```python
from build123d import *

# Parameters (mm, degrees)
F0_W      = 1625
F0_H      = 1960
F1_DEPTH  = 380
F2_W      = 920
F2_H      = 1960
F3_DEPTH  = 228
F4_W      = 1625
F4_H      = 645
F5_DEPTH  = 378
F6_W      = 1480
F6_H      = 185
F7_DEPTH  = 125
F9_DEPTH  = 2
F11_DEPTH = 1
F13_DEPTH = 25
F15_DEPTH = 1625.001


with BuildPart() as f1:
    # F0 (on Top) → F1 (new body)
    with BuildSketch(Plane.XY):
        with Locations((812.5, 980)):
            Rectangle(F0_W, F0_H)
    extrude(amount=F1_DEPTH)

    # F2 (on face) → F3 (cut)
    with BuildSketch(Plane.XY.offset(380)):
        with Locations((808, 980)):
            Rectangle(F2_W, F2_H)
    extrude(amount=-F3_DEPTH, mode=Mode.SUBTRACT)

    # F4 (on face) → F5 (cut)
    with BuildSketch(Plane.XY.offset(380)):
        with Locations((812.5, 1637.5)):
            Rectangle(F4_W, F4_H)
    extrude(amount=-F5_DEPTH, mode=Mode.SUBTRACT)

    # F6 (on face) → F7 (join)
    with BuildSketch(Plane.XY.offset(2)):
        with Locations((812.5, 1407.5)):
            Rectangle(F6_W, F6_H)
    extrude(amount=F7_DEPTH)

    # F8 (on face) → F9 (join)
    with BuildSketch(Plane(origin=(0, 1960, 0), x_dir=(-1, 0, 0), z_dir=(0, 1, 0))):
        with BuildLine():
            Line((-1625, 1126), (-1625, 0))
            Line((-1625, 0), (0, 0))
            Line((0, 0), (0, 1126))
            ThreePointArc((0, 1126), (-58.578644, 1267.421356), (-200, 1326))
            Line((-200, 1326), (-1425, 1326))
            ThreePointArc((-1425, 1326), (-1566.421356, 1267.421356), (-1625, 1126))
        make_face()
    extrude(amount=F9_DEPTH)

    # F10 (on face) → F11 (join)
    with BuildSketch(Plane.XZ):
        with BuildLine():
            Line((0, 1126), (0, 0))
            Line((0, 0), (1625, 0))
            Line((1625, 0), (1625, 1126))
            ThreePointArc((1625, 1126), (1566.421356, 1267.421356), (1425, 1326))
            Line((1425, 1326), (200, 1326))
            ThreePointArc((200, 1326), (58.578644, 1267.421356), (0, 1126))
        make_face()
    extrude(amount=F11_DEPTH)

    # F12 (on face) → F13 (cut)
    with BuildSketch(Plane.XZ.offset(1)):
        with BuildLine():
            Line((358, 1120), (358, 150))
            Line((358, 150), (1258, 150))
            Line((1258, 150), (1258, 1120))
            ThreePointArc((1258, 1120), (1228.710678, 1190.710678), (1158, 1220))
            Line((1158, 1220), (458, 1220))
            ThreePointArc((458, 1220), (387.289322, 1190.710678), (358, 1120))
        make_face()
    extrude(amount=-F13_DEPTH, mode=Mode.SUBTRACT)

    # F14 (on face) → F15 (cut, through all)
    with BuildSketch(Plane.YZ.offset(1625)):
        Polygon((1315, 380), (1055, 380), (1315, 152), align=None)
    extrude(amount=-F15_DEPTH, mode=Mode.SUBTRACT)


solid = f1.part
```
Design review of the part built by this model. Coordinates are the model's own, in mm. A direction names the side the tool comes from. Coordinates: 2 decimals unless noted, no trailing zeros. Write each loop counter-clockwise with the first axis right and the second up, starting at its lowest first coordinate (ties: lowest second). Pieces come first, ordered by that corner, then holes.
1) Add section D-D (y = 1377). Write out the cut boundary in (x, z), plus the area to 3 significant figures.
2) Add section C-C (x = 294). Write out the cut boundary in (y, z).
3) Insertion check: pin 1 (5 mm diameter, centred on x = 1420.5, y = 712, fed in from +Z); pin 2 (8 mm diameter, centred on x = 950.5, y = 881, fed in from +Z); pin 3 (1 mm diameter, centred on x = 521.5, z = 915.5, fed in from -Y); pin 4 (20 mm diameter, centred on y = 13.5, z = 650.5, fed in from +X). Each pin has a flat end and moves straight along its axis. Give the tip position at first contact, or say it passes through.
4) Machinability: for faces 1 (the flat face through (824, 1960, 673)), 2 (the flat face through (72.5, 1406, 64)), 3 (the cylindrical face through (1567.968, -0.493, 1265.858)), 4 (the flat face through (1268, 648, 268)), 5 (the flat face through (1552.5, 1406, 64)), which of the approach directions +Z, -Z, +X, -X, +Y, -Y give a long, thin tool a straight path to every point of the face, cutting with its end or side? Answer none if there is none.
5) Add section B-B (x = 828). Write out the cut boundary in (y, z).
6) Mouldability with a two-part tool opening along Z and no side actions: class faces 6 (the flat face through (802, 1500, 64)), 7 (the flat face through (801, 994, 0)), 8 (the cylindrical face through (57.032, 1960.986, 1265.858)), 9 (the cylindrical face through (1229.484, -0.507, 1189.929)) as +Z half, -Z half, draft (parallel to the pull), parting line (faces both ways), or undercut.
7) To check wall thickness, follow L1, parallel to X at y = 213.5, z = 313; L2, parallel to Y at x = 1550, z = 1160; L3, parallel to Z at x = 596, y = 606. State the ranges of each line that lie inside material, in increasing order.
8) Add section A-A (z = 683). Write out the cut boundary in (x, y).
Check result:
1. outline: (0, 0) - (1625, 0) - (1625, 2) - (1552.5, 2) - (1552.5, 127) - (72.5, 127) - (72.5, 2) - (0, 2) - close
1. area: 188,000 mm2
2. outline: (-1, 0) - (1962, 0) - (1962, 1326) - (1960, 1326) - (1960, 2) - (1500, 2) - (1500, 127) - (1315, 127) - (1315, 152) - (1055, 380) - (0, 380) - (0, 1326) - (-1, 1326) - close
3. pin 1: stops at z = 380
3. pin 2: stops at z = 152
3. pin 3: stops at y = 1960
3. pin 4: passes through
4. face 1: +Z, +X, -X
4. face 2: +Z, -X
4. face 3: +Z, +X, +Y, -Y
4. face 4: +Z
4. face 5: +Z, +X
5. outline: (-1, 0) - (1962, 0) - (1962, 1326) - (1960, 1326) - (1960, 2) - (1500, 2) - (1500, 127) - (1315, 127) - (1315, 152) - (24, 152) - (24, 150) - (-1, 150) - close; (-1, 1220) - (0, 1220) - (0, 1326) - (-1, 1326) - close
6. face 6: draft
6. face 7: -Z half
6. face 8: +Z half
6. face 9: undercut
7. L1: x = 0 to 348, 1268 to 1625
7. L2: y = -1 to 0, 1960 to 1962
7. L3: z = 0 to 152
8. outline: (0, -1) - (358, -1) - (358, 0) - (0, 0) - close; (0, 1960) - (1625, 1960) - (1625, 1962) - (0, 1962) - close; (1258, -1) - (1625, -1) - (1625, 0) - (1258, 0) - close
